For this review, use the dimensioned drawing (mm, ordinates from the lowest corner) and the shaded views. A direction names the side the tool comes from. Round coordinates to 2 decimals unless told otherwise and drop trailing zeros. Order: outer loops, then holes, each group sorted by start corner. A loop starts at its lowest first (then second) coordinate and runs counter-clockwise, first axis right, second up. Notation, with made-up numbers: M 46.25,-35 L 80.25,-35 A22 cw 80.25,2 Z; hole C 61.25,15 d6. An arc over 180 degrees is marked long. Put each result on its own line as item: value.
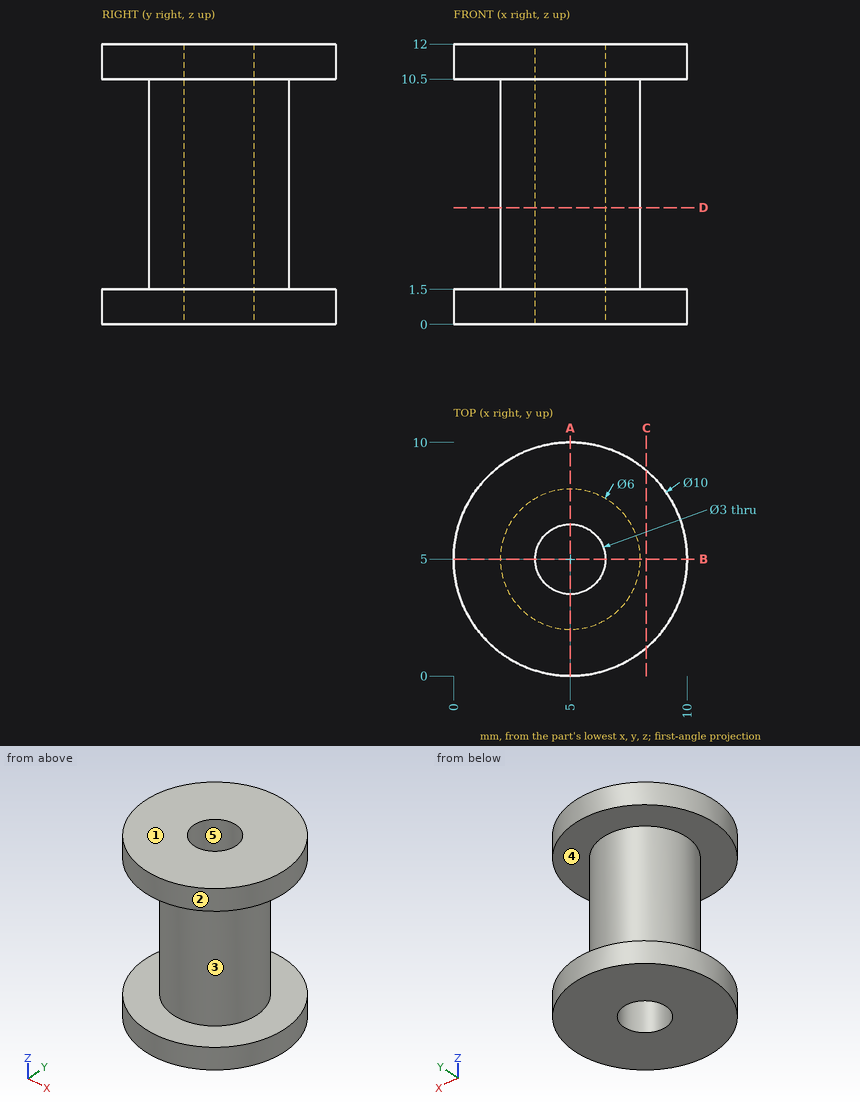
(1) Insertion check: pin 1 Ø1.5 at (y, z) = (8, 2.5) entering from +X; pin 2 Ø1.8 at (x, y) = (5, 5) entering from -Z; pin 3 Ø4 at (x, z) = (4, 5.5) entering from -Y; pin 4 Ø5 at (y, z) = (2.5, 7) entering from +X. Each pin has a flat end and moves straight along its axis. Give the tip position at first contact, or say it passes through.
A:
pin 1: stops at x = 6.98
pin 2: passes through
pin 3: stops at y = 2
pin 4: stops at x = 8
(2) Add section C-C on x = 8.25. Give the boundary of the cut face in (y, z), then the cut area to 3 significant figures.
A:
outline: M 1.2,0 L 8.8,0 L 8.8,1.5 L 1.2,1.5 Z; M 1.2,10.5 L 8.8,10.5 L 8.8,12 L 1.2,12 Z
area: 22.8 mm2
(3) Add section A-A on x = 5. Give the boundary of the cut face in (y, z), then the cut area to 3 significant figures.
A:
outline: M 0,0 L 3.5,0 L 3.5,12 L 0,12 L 0,10.5 L 2,10.5 L 2,1.5 L 0,1.5 Z; M 6.5,0 L 10,0 L 10,1.5 L 8,1.5 L 8,10.5 L 10,10.5 L 10,12 L 6.5,12 Z
area: 48.0 mm2
(4) To check wall thickness, follow L1, parallel to Y at x = 5, z = 2.75; L2, parallel to Z at x = 3.5, y = 1.25; L3, parallel to X at y = 6, z = 9.75. State the ranges of each line that lie inside material, in increasing order.
A:
L1: y = 2 to 3.5, 6.5 to 8
L2: z = 0 to 1.5, 10.5 to 12
L3: x = 2.17 to 3.88, 6.12 to 7.83
(5) For the marked faces 4 and 5, list the 3-axis set-ups (+Z, -Z, +X, -X, +Y, -Y) from which the entire face can be reached by the end or side of a thin tool; tool diameter is ignored.
A:
face 4: none
face 5: +Z, -Z
(6) Add section D-D on z = 5. Give the boundary of the cut face in (x, y).
A:
outline: C 5,5 d6; hole C 5,5 d3
(7) Draft analysis for pull direction Z (two halves, no side actions). For the marked faces 1, 2 and 3, state which applies: released by +Z, released by -Z, zero draft, split by the parting line, or undercut.
A:
face 1: released by +Z
face 2: zero draft
face 3: undercut
